Could you check a few things on this drawing? It's one solid part, dimensions in mm from its lowest x, y, z. A direction names the side the tool comes from. Give positions to 0.01 mm unless a question says otherwise; leave off trailing zeros. Order: outer loops, then holes, each group sorted by start corner. A loop starts at its lowest first (then second) coordinate and runs counter-clockwise, first axis right, second up. Notation, with made-up numbers: M 83.5,85.5 L 96.5,85.5 A18 ccw 96.5,97.5 Z; hole C 86,-23.5 d9. An arc over 180 degrees is marked long. One line per item, written item: value. Start each with the question number.
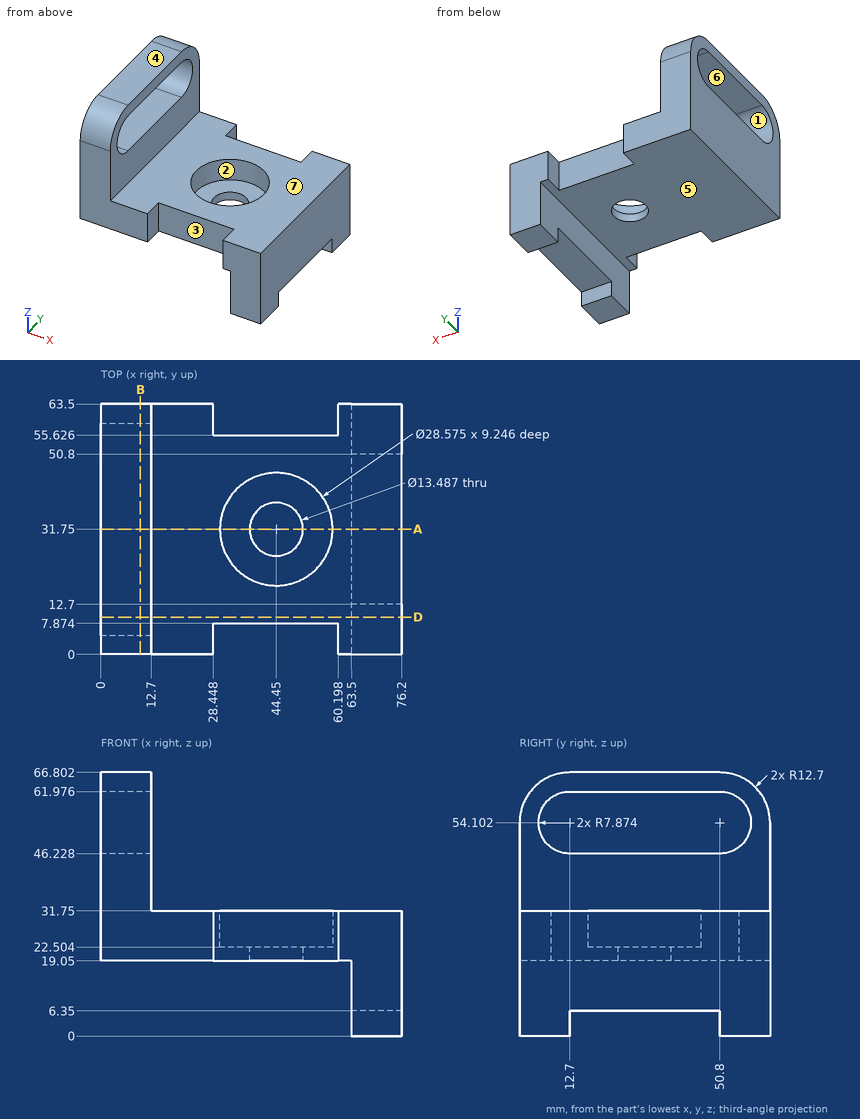
Item 1: I want a section at A-A on y = 31.75. Count the separate pieces of the cut face and the enclosed holes in it, plus the area to 3 significant figures.
Item 2: For the marked faces 5, 6 and 7, which set-ups out of +Z, -Z, +X, -X, +Y, -Y let a thin tool reach every point of the face, with its end or its side?
Item 3: Will these pins go through, and if not, where does the flat tip stop? P1, Ø1.5, axis at x = 18, y = 8, coming from the +Z side; P2, Ø6.5, axis at x = 51.5, z = 28, coming from the +Y side; P3, Ø21, axis at y = 19.5, z = 6, coming from the -X side; P4, Ø8, axis at x = 44.45, y = 31.75, coming from the +Z side.
Item 4: I want a section at D-D on y = 9.5. Write out the boundary of the cut face in (x, z), plus the area to 3 significant figures.
Item 5: I want a section at B-B on x = 10. Write out the boundary of the cut face in (y, z), plus the area to 3 significant figures.
Item 6: Please list where these lines run through material, in increasing order: probe 1 along Z at (x, y) = (5, 46); probe 2 along Y at (x, z) = (44.45, 25.5); probe 3 along X at (y, z) = (31, 26). Write a range as [from, to].
Item 7: We'd pull the mould along Y, two halves only. Please class the marked faces 1, 2, 3 and 4: +Y half, -Y half, draft (parallel to the pull), parting line (faces both ways), or undercut.
Answer below:
1. separate pieces: 3
1. enclosed holes: 0
1. area: 1,060 mm²
2. face 5: -Z, -X, +Y, -Y
2. face 6: +X, -X
2. face 7: +Z, +X, +Y, -Y
3. P1: stops at z = 31.75
3. P2: stops at y = 55.63
3. P3: stops at x = 63.5
3. P4: passes through
4. outline: M 0,19.05 L 63.5,19.05 L 63.5,0 L 76.2,0 L 76.2,31.75 L 12.7,31.75 L 12.7,46.91 L 0,46.91 Z; M 0,61.3 L 12.7,61.3 L 12.7,66.39 L 0,66.39 Z
4. area: 1,470 mm²
5. outline: M 0,19.05 L 63.5,19.05 L 63.5,54.1 A12.7 ccw 50.8,66.8 L 12.7,66.8 A12.7 ccw 0,54.1 Z; hole M 12.7,46.23 L 50.8,46.23 A7.87 ccw 50.8,61.98 L 12.7,61.98 A7.87 ccw Z
5. area: 2,170 mm²
6. probe 1: z = [19.05, 46.23], [61.98, 66.8]
6. probe 2: y = [7.87, 17.46], [46.04, 55.63]
6. probe 3: x = [0, 30.18], [58.72, 76.2]
7. face 1: undercut
7. face 2: undercut
7. face 3: -Y half
7. face 4: draft
